Input: part model. Units: mm. Frame: model coordinates. A direction names the side the tool comes from. Coordinates: 2 decimals unless noted, no trailing zeros. Loops run counter-clockwise (first coordinate to the right, second up) from the corner with the lowest first, then second, coordinate; pieces in that order, holes last.
Item 1: Section B-B on z = 1.25. Give the number of separate pieces and of enclosed holes in the cut face, and give its area (3 significant figures).
Item 2: Section D-D on x = -33.5. Return loops of the section in (y, z).
Item 3: Contact query for flat-ended pins moving along their axis: P1, Ø17, axis at x = 0, y = 0, coming from the +Z side; P2, Ø1.5, axis at x = 26, z = 4, coming from the -Y side; P3, Ø1, axis at x = -1, z = 2.5, coming from the -Y side; P4, Ø1, axis at y = -19.5, z = 1.5, coming from the +X side. Output: stop coordinate, or through.
Item 4: Section A-A on y = 0. Return loops of the section in (x, z), and give its area (3 significant figures).
Item 5: Pull-direction query (Y, two-part tool) for faces 3 (the cylindrical face through (-38.646, -6.753, 3.451)), 4 (the cylindrical face through (25.17, -30.09, 3.45)), 5 (the flat face through (22.16, -9.7, 3.45)), 6 (the flat face through (-2.6, 34.9, 3.5)); classes: released by +Y, released by -Y, zero draft, split by the parting line, or undercut.
Item 6: Section C-C on y = 13.5. Return loops of the section in (x, z), and give its area (3 significant figures).
Item 7: Ray query, line 1 along Y through (x, z) = (0, 2.25); line 2 along X through (y, z) = (-11.5, 2.5); line 3 along X through (y, z) = (10, 2.5). Return the intervals inside material, ascending.
Item 8: Reachability of faces 1 (the cylindrical face through (41.73, -10.57, 3.45)), 2 (the flat face through (-2.68, 24.04, 3.45)) from +Z, -Z, +X, -X, +Y, -Y: full face, straight path, thin tool, end or side. Return the list, or none.
```python
from build123d import *

# Parameters (mm, degrees)
F0_R     = 9.45
F1_DEPTH = 7


with BuildPart() as f1:
    # F0 (on Top) → F1 (new body)
    with BuildSketch(Plane.XY):
        with BuildLine():
            ThreePointArc((-24.555476, 10.805503), (-38.89385, -6.957617), (-59.095755, -17.587779))
            ThreePointArc((-59.095755, -17.587779), (-29.547878, -30.85808), (0, -17.587779))
            ThreePointArc((0, -17.587779), (0.616641, -22.365553), (-3.718256, -24.466991))
            ThreePointArc((-3.718256, -24.466991), (-0.778036, -26.710105), (2.919898, -26.668418))
            ThreePointArc((2.919898, -26.668418), (25.472398, -30.204253), (44.779341, -42.384536))
            ThreePointArc((44.779341, -42.384536), (41.49782, -10.160173), (15.231463, 8.79389))
            ThreePointArc((15.231463, 8.79389), (19.060817, 11.716804), (23.048163, 9.013391))
            ThreePointArc((23.048163, 9.013391), (23.520647, 12.681254), (21.635578, 15.862915))
            ThreePointArc((21.635578, 15.862915), (13.421452, 37.16187), (14.316414, 59.972315))
            ThreePointArc((14.316414, 59.972315), (-11.949942, 41.018252), (-15.231463, 8.79389))
            ThreePointArc((-15.231463, 8.79389), (-19.677458, 10.64875), (-19.329907, 15.453599))
            ThreePointArc((-19.329907, 15.453599), (-22.742611, 14.028851), (-24.555476, 10.805503))
        make_face()
        Polygon((-25.88408, -21.526539), (-32.098543, -17.792513), (-31.972013, -10.543617), (-25.63102, -7.028748), (-19.416557, -10.762774), (-19.543087, -18.011669), align=None, mode=Mode.SUBTRACT)
        Circle(F0_R, mode=Mode.SUBTRACT)
        Polygon((31.58457, -11.653002), (31.45804, -18.901897), (25.117047, -22.416767), (18.902584, -18.682741), (19.029114, -11.433845), (25.370107, -7.918976), align=None, mode=Mode.SUBTRACT)
        Polygon((-5.70049, 33.179541), (0.640503, 36.69441), (6.854966, 32.960384), (6.728436, 25.711489), (0.387443, 22.196619), (-5.82702, 25.930645), align=None, mode=Mode.SUBTRACT)
    extrude(amount=F1_DEPTH)


solid = f1.part
```
Results found:
1. separate pieces: 1
1. enclosed holes: 4
1. area: 3,810 mm2
2. outline: (-30.66, 0) - (-1.9, 0) - (-1.9, 7) - (-30.66, 7) - close
3. P1: passes through
3. P2: stops at y = -30.7
3. P3: stops at y = -26.79
3. P4: stops at x = 45.53
4. outline: (-31.81, 0) - (-9.45, 0) - (-9.45, 7) - (-31.81, 7) - close; (9.45, 0) - (33.09, 0) - (33.09, 7) - (9.45, 7) - close
4. area: 322 mm2
5. face 3: released by +Y
5. face 4: released by -Y
5. face 5: undercut
5. face 6: undercut
6. outline: (-23.26, 0) - (-20.23, 0) - (-20.23, 7) - (-23.26, 7) - close; (-16.48, 0) - (23.29, 0) - (23.29, 7) - (-16.48, 7) - close
6. area: 300 mm2
7. line 1: y = -26.91 to -23.22, -17.59 to -9.45, 9.45 to 22.43, 36.34 to 53.9
7. line 2: x = -45.28 to -31.99, -19.43 to 19.03, 31.33 to 42.24
7. line 3: x = -24.98 to -19.18, -15.61 to 15.83, 22.53 to 23.43
8. face 1: +Z, -Z, +X
8. face 2: +Z, -Z
